from build123d import *

# Parameters (mm, degrees)
SKETCH1_R               = 1.5
SKETCH1_R_2             = 3.95
MAIN_BODY_LINK_B1_DEPTH = 21
CUT_EXTRUDE1_REACH      = 170.233
PULLEYIDLER_DEPTH       = 21
FILLET1_R               = 1
SKETCH4_W               = 40.4
SKETCH4_H               = 7.4
SKETCH4_W_2             = 38.1446978
SKETCH4_H_2             = 45.516821784
CUT_EXTRUDE2_DEPTH      = 169.23348591
CUT_EXTRUDE4_DEPTH      = 124.656147707


with BuildPart() as part:
    # Sketch1 → Main Body Link B1 (new body)
    with BuildSketch(Plane.XY):
        with BuildLine():
            Line((0, 83.474052381), (9.1, 83.474052381))
            Line((9.1, 83.474052381), (9.1, 89.474052381))
            Line((9.1, 89.474052381), (11.1, 89.474052381))
            Line((11.1, 89.474052381), (11.1, 83.474052381))
            Line((11.1, 83.474052381), (20.2, 83.474052381))
            Line((20.2, 83.474052381), (20.2, 90.874052381))
            Line((20.2, 90.874052381), (17.986683974, 148.383116621))
            ThreePointArc((17.986683974, 148.383116621), (0, 165.690874165), (-17.986683974, 148.383116621))
            Line((-17.986683974, 148.383116621), (-20.2, 90.874052381))
            Line((-20.2, 90.874052381), (-20.2, 83.474052381))
            Line((-20.2, 83.474052381), (-11.1, 83.474052381))
            Line((-11.1, 83.474052381), (-11.1, 89.474052381))
            Line((-11.1, 89.474052381), (-9.1, 89.474052381))
            Line((-9.1, 89.474052381), (-9.1, 83.474052381))
            Line((-9.1, 83.474052381), (0, 83.474052381))
        make_face()
        with Locations(Location((5.2, 88.124052381, 0), (0, 0, 180))):
            Circle(SKETCH1_R, mode=Mode.SUBTRACT)
        with Locations(Location((15, 88.124052381, 0), (0, 0, 180))):
            Circle(SKETCH1_R, mode=Mode.SUBTRACT)
        with Locations(Location((-15, 88.124052381, 0), (0, 0, 180))):
            Circle(SKETCH1_R, mode=Mode.SUBTRACT)
        with Locations(Location((-5.2, 88.124052381, 0), (0, 0, 180))):
            Circle(SKETCH1_R, mode=Mode.SUBTRACT)
        with Locations(Location((0, 147.690874165, 0), (0, 0, 180))):
            Circle(SKETCH1_R_2, mode=Mode.SUBTRACT)
    extrude(amount=MAIN_BODY_LINK_B1_DEPTH)

    # Sketch2 → Cut-Extrude1 (cut, up to next)
    with BuildSketch(Plane.XY.offset(21), mode=Mode.PRIVATE) as cut_extrude1_sk1:
        Polygon((-3.278172542, 117.482670232), (12, 128.172168466), (12, 106.793171999), align=None)
    cut_extrude1_tool1 = extrude(cut_extrude1_sk1.sketch, amount=-CUT_EXTRUDE1_REACH, mode=Mode.PRIVATE) & part.part
    # Sketch2 → Cut-Extrude1 (cut, up to next)
    with BuildSketch(Plane.XY.offset(21), mode=Mode.PRIVATE) as cut_extrude1_sk2:
        with BuildLine():
            ThreePointArc((-12, 134.2744663), (-7.774454217, 131.456408925), (-2.929911079, 129.930929878))
            Line((-2.929911079, 129.930929878), (-12, 123.584968066))
            Line((-12, 123.584968066), (-12, 134.2744663))
        make_face()
    cut_extrude1_tool2 = extrude(cut_extrude1_sk2.sketch, amount=-CUT_EXTRUDE1_REACH, mode=Mode.PRIVATE) & part.part
    # Sketch2 → Cut-Extrude1 (cut, up to next)
    with BuildSketch(Plane.XY.offset(21), mode=Mode.PRIVATE) as cut_extrude1_sk3:
        Polygon((-12, 111.380372399), (-12, 100.690874165), (3.278172542, 100.690874165), align=None)
    cut_extrude1_tool3 = extrude(cut_extrude1_sk3.sketch, amount=-CUT_EXTRUDE1_REACH, mode=Mode.PRIVATE) & part.part
    add(cut_extrude1_tool1.solids().sort_by_distance((6.907276, 117.48267, 21))[0], mode=Mode.SUBTRACT)
    add(cut_extrude1_tool2.solids().sort_by_distance((-9.12997, 128.978342, 21))[0], mode=Mode.SUBTRACT)
    add(cut_extrude1_tool3.solids().sort_by_distance((-6.907276, 104.25404, 21))[0], mode=Mode.SUBTRACT)

    # Sketch3 → PulleyIdler (cut)
    with BuildSketch(Plane.XY.offset(21)):
        with BuildLine():
            Line((-5.959092644, 108.984491566), (6.331359583, 100.385376259))
            ThreePointArc((6.331359583, 100.385376259), (11.205592008, 101.246688207), (10.34428006, 106.120920631))
            Line((10.34428006, 106.120920631), (-1.946172167, 114.720035938))
            ThreePointArc((-1.946172167, 114.720035938), (-6.820404592, 113.85872399), (-5.959092644, 108.984491566))
        make_face()
    extrude(amount=-PULLEYIDLER_DEPTH, mode=Mode.SUBTRACT)

    # Fillet1
    fillet1_edges = [part.edges().sort_by_distance(p)[0] for p in [
        (-3.278172542, 117.482670232, 10.5),
        (12, 128.172168466, 10.5),
        (12, 106.793171999, 10.5),
        (-12, 134.2744663, 10.5),
        (-2.929911079, 129.930929878, 10.5),
        (-12, 123.584968066, 10.5),
        (-12, 111.380372399, 10.5),
        (3.278172542, 100.690874165, 10.5),
        (-12, 100.690874165, 10.5),
    ]]
    fillet(fillet1_edges, radius=FILLET1_R)

    # Sketch4 → Cut-Extrude2 (cut, through all)
    with BuildSketch(Plane.XY.offset(21)):
        with Locations((0, 87.174052381)):
            Rectangle(SKETCH4_W, SKETCH4_H)
        with Locations((0, 142.932463273)):
            Rectangle(SKETCH4_W_2, SKETCH4_H_2)
    extrude(amount=-CUT_EXTRUDE2_DEPTH, mode=Mode.SUBTRACT)

    # Sketch5 → Cut-Extrude4 (cut, through all)
    with BuildSketch(Plane.XY.offset(21)):
        with BuildLine():
            Line((-12, 100.690874165), (5.894720779, 100.690874165))
            Line((5.894720779, 100.690874165), (6.331359583, 100.385376259))
            ThreePointArc((6.331359583, 100.385376259), (8.580755157, 99.761589707), (10.722091306, 100.690874165))
            Line((10.722091306, 100.690874165), (12, 100.690874165))
            Line((12, 100.690874165), (12, 120.174052381))
            Line((12, 120.174052381), (-12, 120.174052381))
            Line((-12, 120.174052381), (-12, 100.690874165))
        make_face()
    extrude(amount=-CUT_EXTRUDE4_DEPTH, mode=Mode.SUBTRACT)


solid = part.part
The listing builds one solid part. Answer for the finished solid, in the listing's coordinates (mm). A direction names the side the tool comes from. Give positions to 0.01 mm unless a question says otherwise; leave off trailing zeros. Write each loop counter-clockwise with the first axis right and the second up, starting at its lowest first coordinate (ties: lowest second). Pieces come first, ordered by that corner, then holes.
1) Given P1, Ø6, axis at x = -7, y = 114, coming from the -Z side; P2, Ø1.5, axis at y = 113.5, z = 18.5, coming from the +X side; P3, Ø9, axis at x = -6, z = 11.5, coming from the +Y side; P4, Ø9.5, axis at y = 110.5, z = 8.5, coming from the +X side, each flat-ended and moving along its own axis, determine where each tip first touches the part or whether it passes through.
2) Section A-A (z = 11.75) is taken. Write down the section's boundary in (x, y).
3) Section C-C (x = -6.5) is taken. Write down the section's boundary in (y, z), and give its area (3 significant figures).
4) Section B-B (y = 113.25) is taken. Write down the section's boundary in (x, z).
5) A tool of negligible diameter and unlimited length cuts with its end or side. For faces 5 (the face through (15, 120.174, 11)), 6 (the face through (-12, 111, 11)), from which of +Z, -Z, +X, -X, +Y, -Y can it reach the whole face along a straight path? Write none if from no direction.
6) Section D-D (y = 104) is taken. Write down the section's boundary in (x, z), and give its area (3 significant figures).
7) Find the intervals of material crossed by L1, parallel to X at y = 107.25, z = 10.25; L2, parallel to X at y = 118, z = 13.75; L3, parallel to Y at x = -7, z = 18.5, in increasing order.
8) For a pull along X with two mould halves and no side action, classify faces 1 (the face through (11, 100.691, 11)), 2 (the face through (-19.63, 105.73, 10.35)), 3 (the face through (-16, 120.174, 11)), 4 (the face through (-3, 100.691, 11)) as pulls with the +X half, pulls with the -X half, needs draft (parallel to the pull), parting line crosses it, or undercut.
Response:
1. P1: passes through
1. P2: stops at x = 19.36
1. P3: stops at y = 100.69
1. P4: stops at x = 19.63
2. outline: (-20.2, 90.87) - (20.2, 90.87) - (19.07, 120.17) - (12, 120.17) - (12, 100.69) - (10.72, 100.69) arc R3.5 cw to (6.33, 100.39) - (5.89, 100.69) - (-12, 100.69) - (-12, 120.17) - (-19.07, 120.17) - close
3. outline: (90.87, 0) - (100.69, 0) - (100.69, 21) - (90.87, 21) - close
3. area: 206 mm2
4. outline: (-19.34, 0) - (-12, 0) - (-12, 21) - (-19.34, 21) - close; (12, 0) - (19.34, 0) - (19.34, 21) - (12, 21) - close
5. face 5: +Z, -Z, +X, -X, +Y
5. face 6: +Z, -Z, +Y
6. outline: (-19.69, 0) - (-12, 0) - (-12, 21) - (-19.69, 21) - close; (12, 0) - (19.69, 0) - (19.69, 21) - (12, 21) - close
6. area: 323 mm2
7. L1: x = -19.57 to -12, 12 to 19.57
7. L2: x = -19.16 to -12, 12 to 19.16
7. L3: y = 90.87 to 100.69
8. face 1: undercut
8. face 2: pulls with the -X half
8. face 3: needs draft
8. face 4: undercut
